Part model, mm, in its own coordinate system. Give positions to 0.01 mm unless a question says otherwise; leave off trailing zeros. Write each loop counter-clockwise with the first axis right and the second up, starting at its lowest first coordinate (ties: lowest second). Pieces come first, ordered by that corner, then holes.
```python
from build123d import *

# Parameters (mm, degrees)
SKETCH1_W           = 190.5
SKETCH1_H           = 76.2
BOSS_EXTRUDE1_DEPTH = 3.048
SKETCH2_W           = 82.55
SKETCH2_H           = 50.8
SKETCH2_W_2         = 69.85
CUT_EXTRUDE1_DEPTH  = 3.048
SKETCH3_R           = 1.5875
CUT_EXTRUDE2_DEPTH  = 3.048


with BuildPart() as part:
    # Sketch1 → Boss-Extrude1 (new body)
    with BuildSketch(Plane(origin=(0, 0, 0), x_dir=(1, 0, 0), z_dir=(0, 1, 0))):
        with Locations((-95.25, -38.1)):
            Rectangle(SKETCH1_W, SKETCH1_H)
    extrude(amount=BOSS_EXTRUDE1_DEPTH)

    # Sketch2 → Cut-Extrude1 (cut)
    with BuildSketch(Plane(origin=(0, 3.048, 0), x_dir=(1, 0, 0), z_dir=(0, 1, 0))):
        with Locations((-53.975, -38.1)):
            Rectangle(SKETCH2_W, SKETCH2_H)
        with Locations((-142.875, -38.1)):
            Rectangle(SKETCH2_W_2, SKETCH2_H)
    extrude(amount=-CUT_EXTRUDE1_DEPTH, mode=Mode.SUBTRACT)

    # Sketch3 → Cut-Extrude2 (cut)
    with BuildSketch(Plane(origin=(0, 3.048, 0), x_dir=(1, 0, 0), z_dir=(0, 1, 0))):
        with Locations(Location((-6.35, -38.1, 0), (0, 0, 270))):
            Circle(SKETCH3_R)
        with Locations(Location((-184.168238783, -38.1, 0), (0, 0, 270))):
            Circle(SKETCH3_R)
        with Locations(Location((-6.35, -6.35, 0), (0, 0, 270))):
            Circle(SKETCH3_R)
        with Locations(Location((-184.168238783, -6.35, 0), (0, 0, 270))):
            Circle(SKETCH3_R)
        with Locations(Location((-184.168238783, -69.85, 0), (0, 0, 270))):
            Circle(SKETCH3_R)
        with Locations(Location((-6.35, -69.85, 0), (0, 0, 270))):
            Circle(SKETCH3_R)
        with Locations(Location((-19.05, -9.525, 0), (0, 0, 270))):
            Circle(SKETCH3_R)
        with Locations(Location((-19.05, -66.675, 0), (0, 0, 270))):
            Circle(SKETCH3_R)
        with Locations(Location((-141.9225, -9.525, 0), (0, 0, 270))):
            Circle(SKETCH3_R)
        with Locations(Location((-141.9225, -66.675, 0), (0, 0, 270))):
            Circle(SKETCH3_R)
    extrude(amount=-CUT_EXTRUDE2_DEPTH, mode=Mode.SUBTRACT)


solid = part.part
```
1) Wall check: L1, parallel to X at y = 0.8, z = 41.5; L2, parallel to X at y = 1.7, z = 38.1; L3, parallel to X at y = 1.65, z = 69.85. Give the ranges that are in metal, low to high.
Answers follow:
L1: x = -190.5 to -177.8, -107.95 to -95.25, -12.7 to 0
L2: x = -190.5 to -185.76, -182.58 to -177.8, -107.95 to -95.25, -12.7 to -7.94, -4.76 to 0
L3: x = -190.5 to -185.76, -182.58 to -7.94, -4.76 to 0
2) Saw through at A-A, the plane z = 34.5. Write the cut outline in (x, y), then the cut area to 3 significant figures.
Answers follow:
outline: (-190.5, 0) - (-177.8, 0) - (-177.8, 3.05) - (-190.5, 3.05) - close; (-107.95, 0) - (-95.25, 0) - (-95.25, 3.05) - (-107.95, 3.05) - close; (-12.7, 0) - (0, 0) - (0, 3.05) - (-12.7, 3.05) - close
area: 116 mm2
3) Two-plate mould, pull along Z, no slides. Class faces 1 (the face through (-185.72, 1.55, 37.76)), 2 (the face through (-97, 0, 38)): +Z half, -Z half, draft (parallel to the pull), parting line (faces both ways), or undercut.
Answers follow:
face 1: undercut
face 2: draft
4) Pin check, flat tip, straight feed: pin 1 Ø3 at (x, z) = (-19.05, 66.675) entering from +Y. Stop position of the tip, or through.
Answers follow:
pin 1: passes through
5) Saw through at B-B, the plane x = -78. Write the cut outline in (y, z).
Answers follow:
outline: (0, 0) - (3.05, 0) - (3.05, 12.7) - (0, 12.7) - close; (0, 63.5) - (3.05, 63.5) - (3.05, 76.2) - (0, 76.2) - close
6) Saw through at C-C, the plane y = 2. Count the separate pieces of the cut face and the enclosed holes in it, then the cut area to 4 significant figures.
Answers follow:
separate pieces: 1
enclosed holes: 12
area: 6,695 mm2
